Could you check a few things on this model? Use its own coordinates, in mm. A direction names the side the tool comes from. Round coordinates to 2 decimals unless told otherwise and drop trailing zeros. Loops run counter-clockwise (first coordinate to the right, second up) from the corner with the lowest first, then second, coordinate; pieces in that order, holes last. Notation, with made-up numbers: (81, 21.5) - (95, 21.5) arc R6 ccw to (95, 28.5) - close; hole circle Ø11 at (46.25, 1). An arc over 180 degrees is marked (long way). Answer as CSV lines item,"result". Start each with the question number.
1) Suppose I cut it at D-D, the plane x = -29. Write out the boundary of the cut face in (y, z), then the cut area to 3 significant figures.
2) Please list where these lines run through material, in increasing order: line 1 along Y through (x, z) = (0, 7.5); line 2 along Z through (x, y) = (4.5, -7.5); line 3 along Z through (x, y) = (-35, -2.5).
3) Suppose I cut it at A-A, the plane y = 0. Write out the boundary of the cut face in (x, z).
4) Suppose I cut it at C-C, the plane z = -1. Write out the boundary of the cut face in (x, y), then the cut area to 3 significant figures.
5) I'm going to push flat-ended pins straight in: pin 1 Ø6 at (y, z) = (0, 7.5) entering from +X; pin 2 Ø6 at (x, y) = (-39, -0.5) entering from -Z; pin 3 Ø5 at (x, z) = (-7.5, 0) entering from -Y. Where does each tip first touch, or does it pass through?
6) Suppose I cut it at B-B, the plane z = 1.75. Write out the boundary of the cut face in (x, y), then the cut area to 3 significant figures.
7) Which directions (+Z, -Z, +X, -X, +Y, -Y) give clear straight access to the entire face, cutting with the end or side of a thin tool? Please do faces 5 (the face through (8.33, -9.56, -1.52)), 6 (the face through (0.54, -2.44, 7.46)), 7 (the face through (-1, 0, 10)).
8) We'd pull the mould along X, two halves only. Please class faces 1 (the face through (-45, 0, 2)), 2 (the face through (6, -8.1, 0.9)), 3 (the face through (7, -9, -3)), 4 (the face through (0.108, -0.488, 4.93)): pulls with the +X half, pulls with the -X half, needs draft (parallel to the pull), parting line crosses it, or undercut.
```python
from build123d import *

# Parameters (mm, degrees)
SKETCH2_R           = 2.5
BOSS_EXTRUDE1_DEPTH = 5
BOSS_EXTRUDE2_START = -8
SKETCH3_R           = 2.5
SKETCH3_R_2         = 0.5
BOSS_EXTRUDE2_DEPTH = 8
SKETCH4_R           = 2.5
SKETCH4_R_2         = 0.5
BOSS_EXTRUDE3_DEPTH = 10


with BuildPart() as part:
    # Sketch2 → Boss-Extrude1 (new body)
    with BuildSketch(Plane.XY):
        with BuildLine():
            Line((-41, 4), (0, 4))
            ThreePointArc((0, 4), (1.846994453, 3.548043333), (3.276608177, 2.294305745))
            Line((3.276608177, 2.294305745), (9.299160759, -6.30679072))
            ThreePointArc((9.299160759, -6.30679072), (9.389243762, -10.761047968), (5.302836395, -12.53581483))
            Line((5.302836395, -12.53581483), (-41.719716186, -3.934718365))
            ThreePointArc((-41.719716186, -3.934718365), (-44.98364616, 0.361335399), (-41, 4))
        make_face()
        Circle(SKETCH2_R, mode=Mode.SUBTRACT)
        with Locations((6.022552582, -8.601096465)):
            Circle(SKETCH2_R, mode=Mode.SUBTRACT)
    extrude(amount=BOSS_EXTRUDE1_DEPTH)

    # Sketch3 → Boss-Extrude2 (add)
    with BuildSketch(Plane.XY.offset(5).offset(BOSS_EXTRUDE2_START)):
        with Locations((6.022552582, -8.601096465)):
            Circle(SKETCH3_R)
        with Locations((6.022552582, -8.601096465)):
            Circle(SKETCH3_R_2, mode=Mode.SUBTRACT)
    extrude(amount=BOSS_EXTRUDE2_DEPTH)

    # Sketch4 → Boss-Extrude3 (add)
    with BuildSketch(Plane(origin=(0, 0, 0), x_dir=(-1, 0, 0), z_dir=(0, 0, -1))):
        Circle(SKETCH4_R)
        Circle(SKETCH4_R_2, mode=Mode.SUBTRACT)
    extrude(amount=-BOSS_EXTRUDE3_DEPTH)


solid = part.part
```
Filled sheet:
1,outline,"(-6.26, 0) - (4, 0) - (4, 5) - (-6.26, 5) - close"
1,area,"51.3 mm²"
2,line 1,"-2.5 to -0.5, 0.5 to 2.5"
2,line 2,"-3 to 5"
2,line 3,"0 to 5"
3,outline,"(-45, 0) - (-0.5, 0) - (-0.5, 10) - (-2.5, 10) - (-2.5, 5) - (-45, 5) - close; (0.5, 0) - (4.88, 0) - (4.88, 5) - (2.5, 5) - (2.5, 10) - (0.5, 10) - close"
4,outline,"circle Ø5 at (6.02, -8.6); hole circle Ø1 at (6.02, -8.6)"
4,area,"18.8 mm²"
5,pin 1,"x = 6.04"
5,pin 2,"z = 0"
5,pin 3,"y = -10.65"
6,outline,"(-41.72, -3.93) - (5.3, -12.54) arc R4 ccw to (9.3, -6.31) - (3.28, 2.29) arc R4 ccw to (0, 4) - (-41, 4) arc R4 ccw to start; hole circle Ø1 at (0, 0); hole circle Ø1 at (6.02, -8.6)"
6,area,"622 mm²"
7,face 5,"-Z"
7,face 6,"+Z"
7,face 7,"+Z, +X, -X, +Y, -Y"
8,face 1,"pulls with the -X half"
8,face 2,"undercut"
8,face 3,"needs draft"
8,face 4,"undercut"
